```python
from build123d import *

# Parameters (mm, degrees)
F0_R     = 1.5
F1_DEPTH = 3


with BuildPart() as f1:
    # F0 (on Top) → F1 (new body)
    with BuildSketch(Plane.XY):
        with BuildLine():
            Line((-56, 5), (-60, 5))
            Line((-60, 5), (-60, -5))
            Line((-60, -5), (-4.8989794856, -5))
            ThreePointArc((-4.8989794856, -5), (-6.4534043883, -2.7117470016), (-7, 0))
            ThreePointArc((-7, 0), (-6.4534043883, 2.7117470016), (-4.8989794856, 5))
            Line((-4.8989794856, 5), (-52, 5))
            Line((-52, 5), (-52, 3))
            Line((-52, 3), (-56, 3))
            Line((-56, 3), (-56, 5))
        make_face()
        with Locations((-30, 0)):
            Circle(F0_R, mode=Mode.SUBTRACT)
        with BuildLine():
            ThreePointArc((4.8989794856, 5), (0, 7), (-4.8989794856, 5))
            Line((-4.8989794856, 5), (4.8989794856, 5))
        make_face()
        with BuildLine():
            Line((4.8989794856, -5), (-4.8989794856, -5))
            ThreePointArc((-4.8989794856, -5), (0, -7), (4.8989794856, -5))
        make_face()
        with BuildLine():
            ThreePointArc((-7, 0), (-6.4534043883, -2.7117470016), (-4.8989794856, -5))
            Line((-4.8989794856, -5), (4.8989794856, -5))
            ThreePointArc((4.8989794856, -5), (6.4534043883, -2.7117470016), (7, 0))
            ThreePointArc((7, 0), (6.4534043883, 2.7117470016), (4.8989794856, 5))
            Line((4.8989794856, 5), (-4.8989794856, 5))
            ThreePointArc((-4.8989794856, 5), (-6.4534043883, 2.7117470016), (-7, 0))
        make_face()
        with BuildLine():
            ThreePointArc((2, 0), (0, -2), (-2, 0))
            ThreePointArc((-2, 0), (0, 2), (2, 0))
        make_face(mode=Mode.SUBTRACT)
        with BuildLine():
            ThreePointArc((7, 0), (6.4534043883, -2.7117470016), (4.8989794856, -5))
            Line((4.8989794856, -5), (60, -5))
            Line((60, -5), (60, 5))
            Line((60, 5), (59, 5))
            ThreePointArc((59, 5), (53, -1), (47, 5))
            Line((47, 5), (4.8989794856, 5))
            ThreePointArc((4.8989794856, 5), (6.4534043883, 2.7117470016), (7, 0))
        make_face()
        with BuildLine():
            add(Edge.make_bspline(
                [(17.89625742, 2.1835303769), (18.5359551454, 1.5625860049), (18.5359551454, 0.4040454989)],
                knots=[0, 0, 0, 1, 1, 1], degree=2))
            add(Edge.make_bspline(
                [(18.5359551454, 0.4040454989), (18.5359551454, -0.8114496364), (18.1108791324, -1.7081377619)],
                knots=[0, 0, 0, 1, 1, 1], degree=2))
            add(Edge.make_bspline(
                [(18.1108791324, -1.7081377619), (17.6858031194, -2.6048258874), (16.8807980555, -3.0736597253)],
                knots=[0, 0, 0, 1, 1, 1], degree=2))
            add(Edge.make_bspline(
                [(16.8807980555, -3.0736597253), (16.0757929917, -3.5424935631), (14.9811528013, -3.5424935631)],
                knots=[0, 0, 0, 1, 1, 1], degree=2))
            Line((14.9811528013, -3.5424935631), (13.0238583492, -3.5424935631))
            Line((13.0238583492, -3.5424935631), (14.3643758412, 2.8044747489))
            Line((14.3643758412, 2.8044747489), (16.0841278154, 2.8044747489))
            add(Edge.make_bspline(
                [(16.0841278154, 2.8044747489), (17.2565596945, 2.8044747489), (17.89625742, 2.1835303769)],
                knots=[0, 0, 0, 1, 1, 1], degree=2))
        make_face(mode=Mode.SUBTRACT)
        Polygon((22.821443708, -2.4311837252), (22.5866795048, -3.5424935631), (19.0402119844, -3.5424935631), (20.3807294764, 2.8044747489), (23.932753546, 2.8044747489), (23.6979893427, 1.7014997347), (21.4753696668, 1.7014997347), (21.1836508343, 0.3081950254), (23.2548545448, 0.3081950254), (23.0159229297, -0.7947799888), (20.9461083565, -0.7947799888), (20.5988240321, -2.4311837252), align=None, mode=Mode.SUBTRACT)
        Polygon((27.3875380047, -3.5424935631), (27.2833527074, -2.0311121835), (25.2302077818, -2.0311121835), (24.4842410531, -3.5424935631), (23.0951037556, -3.5424935631), (26.4193093084, 2.8308683575), (28.0390433972, 2.8308683575), (28.6766574167, -3.5424935631), align=None, mode=Mode.SUBTRACT)
        with BuildLine():
            Line((35.9668499537, 2.8044747489), (34.6249433244, -3.5424935631))
            Line((34.6249433244, -3.5424935631), (33.1399555534, -3.5424935631))
            Line((33.1399555534, -3.5424935631), (31.5952348786, 1.2583649368))
            Line((31.5952348786, 1.2583649368), (31.56884127, 1.2583649368))
            Line((31.56884127, 1.2583649368), (31.5507824851, 1.1194512071))
            add(Edge.make_bspline(
                [(31.5507824851, 1.1194512071), (31.4118687554, 0.1817835313), (31.2646202019, -0.5558483737)],
                knots=[0, 0, 0, 1, 1, 1], degree=2))
            Line((31.2646202019, -0.5558483737), (30.6353410061, -3.5424935631))
            Line((30.6353410061, -3.5424935631), (29.4420720676, -3.5424935631))
            Line((29.4420720676, -3.5424935631), (30.7825895596, 2.8044747489))
            Line((30.7825895596, 2.8044747489), (32.3328667836, 2.8044747489))
            Line((32.3328667836, 2.8044747489), (33.8081305935, -1.8713613943))
            Line((33.8081305935, -1.8713613943), (33.8261893783, -1.8713613943))
            add(Edge.make_bspline(
                [(33.8261893783, -1.8713613943), (33.8775874583, -1.5407467175), (33.99496956, -0.928831738)],
                knots=[0, 0, 0, 1, 1, 1], degree=2))
            add(Edge.make_bspline(
                [(33.99496956, -0.928831738), (34.1123516616, -0.3169167585), (34.7763592898, 2.8044747489)],
                knots=[0, 0, 0, 1, 1, 1], degree=2))
            Line((34.7763592898, 2.8044747489), (35.9668499537, 2.8044747489))
        make_face(mode=Mode.SUBTRACT)
    extrude(amount=F1_DEPTH)


solid = f1.part
```
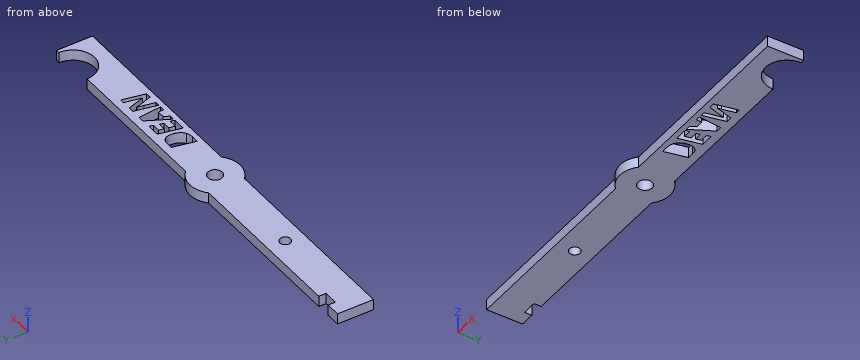
Model file for the job. Use its own axes, mm. Round coordinates to 2 decimals unless told otherwise and drop trailing zeros. Write each loop counter-clockwise with the first axis right and the second up, starting at its lowest first coordinate (ties: lowest second). Pieces come first, ordered by that corner, then holes. Notation, with made-up numbers: (68, 58.5) -> (124, 58.5) arc R17 cw to (124, 73.5) -> close; hole circle Ø6 at (68, -37.75). An arc over 180 degrees is marked (long way). Answer as CSV lines item,"result".
1. Slice it at D-D, the plane x = -30. List the corners of the cut face in (y, z).
Resolved:
outline,"(-5, 0) -> (-1.5, 0) -> (-1.5, 3) -> (-5, 3) -> close; (1.5, 0) -> (5, 0) -> (5, 3) -> (1.5, 3) -> close"
2. Slice it at B-B, the plane z = 0.75. State how many separate pieces and enclosed holes the cut face has, plus the area to 3 significant figures.
Resolved:
separate pieces,"1"
enclosed holes,"6"
area,"1,060 mm²"
3. Slice it at C-C, the plane x = 53. List the corners of the cut face in (y, z), plus the area to 3 significant figures.
Resolved:
outline,"(-5, 0) -> (-1, 0) -> (-1, 3) -> (-5, 3) -> close"
area,"12.0 mm²"
4. Slice it at A-A, the plane x = 0. List the corners of the cut face in (y, z), plus the area to 3 significant figures.
Resolved:
outline,"(-7, 0) -> (-2, 0) -> (-2, 3) -> (-7, 3) -> close; (2, 0) -> (7, 0) -> (7, 3) -> (2, 3) -> close"
area,"30.0 mm²"
5. Pin check, flat tips, straight feed: pin 1 Ø1.5 at (x, z) = (-57, 1) entering from +Y; pin 2 Ø1.5 at (x, z) = (-44.5, 1.5) entering from -Y; pin 3 Ø1.5 at (x, z) = (1.5, 0.5) entering from -Y; pin 4 Ø4 at (x, y) = (-30, 0) entering from +Z. Stop position of each tip, or through.
Resolved:
pin 1,"y = 5"
pin 2,"y = -5"
pin 3,"y = -6.96"
pin 4,"z = 3"
6. Drill centre lines: line 1 (Y direction, x = -30, z = 2.25); line 2 (Y direction, x = 16.5, z = 2.55); line 3 (Y direction, x = 41, z = 0.2). Where is each one in solid material? Low to high.
Resolved:
line 1,"-5 to -1.5, 1.5 to 5"
line 2,"-5 to -3.26, 2.78 to 5"
line 3,"-5 to 5"
